Autodesk Inventor part; units mm, degrees
ref_plane "YZ Plane" through (0, 0, 0) normal (1, 0, 0) x (0, 1, 0)
ref_plane "XZ Plane" through (0, 0, 0) normal (0, 1, 0) x (-1, 0, 0)
ref_plane "XY Plane" through (0, 0, 0) normal (0, 0, 1) x (1, 0, 0)
sketch "Sketch1" plane through (0, 0, 0) normal (0, 0, 1) x (1, 0, 0)
  circle A0 centre (0, 0) radius 6.94 construction
  circle A1 centre (0, 0) radius 6.93
  point P0 (0, 0)
  dimension "d0" = 0.01
sketch "Sketch1 outline for Extrusion1" plane through (0, 0, 0) normal (0, 0, 1) x (1, 0, 0)
  circle A0 centre (0, 0) radius 6.93
extrude "Extrusion1" add sketch "Sketch1 outline for Extrusion1" against normal blind 20
sketch "Sketch2" plane through (0, 0, 0) normal (1, 0, 0) x (0, 1, 0)
  line L0 (-6.93, -20) -> (6.93, -20) construction
  line L1 (-6.93, 0) -> (6.93, 0) construction
  line L2 (6.93, -20) -> (6.93, -1.5)
  line L3 (6.93, -1.5) -> (5.93, -20)
  line L4 (6.93, -20) -> (5.93, -20)
  line L5 (0, 4) -> (0, -24)
  point P0 (0, 0)
  dimension "d3" = 1.5
  dimension "d4" = 1
sketch "Sketch2 outline for Revolution1" plane through (0, 0, 0) normal (1, 0, 0) x (0, 1, 0)
  line L0 (5.93, -20) -> (6.93, -20)
  line L1 (6.93, -1.5) -> (5.93, -20)
  line L2 (6.93, -20) -> (6.93, -1.5)
revolve "Revolution1" cut sketch "Sketch2 outline for Revolution1" angle 360 about axis through (0, 0, 0) along (0, 0, -1)
sketch "Sketch3" plane through (0, 0, 0) normal (0, 0, 1) x (1, 0, 0)
  circle A0 centre (0, 0) radius 6.93 construction
  circle A1 centre (0, 0) radius 14.43
  dimension "d6" = 7.5
sketch "Sketch3 outline for Extrusion2" plane through (0, 0, 0) normal (0, 0, 1) x (1, 0, 0)
  circle A0 centre (0, 0) radius 14.43
extrude "Extrusion2" add sketch "Sketch3 outline for Extrusion2" along normal blind 1.5
sketch "Sketch4" plane through (0, 0, -20) normal (0, 0, -1) x (-1, 0, 0)
  circle A0 centre (0, 0) radius 5.93 construction
  circle A1 centre (0, 0) radius 4.43
  dimension "d9" = 1.5
sketch "Sketch4 outline for Extrusion3" plane through (0, 0, -20) normal (0, 0, -1) x (-1, 0, 0)
  circle A0 centre (0, 0) radius 4.43
extrude "Extrusion3" cut sketch "Sketch4 outline for Extrusion3" against normal through all
sketch "Sketch5" plane through (0, 0, 0) normal (1, 0, 0) x (0, 1, 0)
  line L0 (-4.43, 1.5) -> (4.43, 1.5) construction
  line L1 (14.43, 1.5) -> (-14.43, 1.5) construction
  line L2 (4.43, 1.5) -> (14.43, 1.5)
  line L3 (14.43, 1.5) -> (14.43, 18.820508)
  line L4 (14.43, 18.820508) -> (4.43, 1.5)
  point P0 (0, 0)
  dimension "d15" = 60
sketch "Sketch5 outline for Extrusion4" plane through (0, 0, 0) normal (1, 0, 0) x (0, 1, 0)
  line L0 (14.43, 18.820508) -> (4.43, 1.5)
  line L1 (14.43, 1.5) -> (14.43, 18.820508)
  line L2 (4.43, 1.5) -> (14.43, 1.5)
extrude "Extrusion4" add sketch "Sketch5 outline for Extrusion4" along normal mid plane 8
ref_plane "Work Plane1" through (0, 4.43, 1.5) normal (0, 0.5, 0.8660254) x (-1, 0, 0)
sketch "Sketch6" plane through (-4, 14.43, 18.820508) normal (0, -0.8660254, 0.5) x (1, 0, 0)
  line L0 (0, -20) -> (0, 0)
  line L1 (0.50115, -8.72775) -> (7.50139, -8.72775)
  line L2 (8, -20) -> (0, -20)
  line L3 (0, -20) -> (0, -8.97775)
  line L4 (0, -8.97775) -> (8, -8.97775)
  line L5 (8, -8.97775) -> (8, -20)
  point P0 (4, -23.514038)
  dimension "d16" = 0.25
sketch "Sketch6 outline for Extrusion5" plane through (-4, 14.43, 18.820508) normal (0, -0.8660254, 0.5) x (1, 0, 0)
  line L0 (0, -20) -> (8, -20)
  line L1 (0, -8.97775) -> (0, -20)
  line L2 (8, -8.97775) -> (0, -8.97775)
  line L3 (8, -20) -> (8, -8.97775)
extrude "Extrusion5" add sketch "Sketch6 outline for Extrusion5" along normal blind 0.5
sketch "Sketch7" plane through (4, 0, 0) normal (1, 0, 0) x (0, 0, -1)
  line L0 (-1.5, 14.43) -> (-18.820508, 14.43) construction
  line L1 (-18.820508, 14.43) -> (-11.045549, 9.941125) construction
  line L2 (-18.820508, 14.43) -> (-14.820508, 14.43)
  line L3 (-18.820508, 14.43) -> (-14.820508, 12.120599)
  line L4 (-14.820508, 14.43) -> (-14.820508, 12.120599)
  point P0 (0, 0)
  dimension "d19" = 4
sketch "Sketch7 outline for Extrusion6" plane through (4, 0, 0) normal (1, 0, 0) x (0, 0, -1)
  line L0 (-18.820508, 14.43) -> (-14.820508, 14.43)
  line L1 (-14.820508, 14.43) -> (-14.820508, 12.120599)
  line L2 (-14.820508, 12.120599) -> (-18.820508, 14.43)
extrude "Extrusion6" cut sketch "Sketch7 outline for Extrusion6" against normal up to surface (8 mm away)
sketch "Sketch8" plane through (0, 0, 0) normal (0, 0, -1) x (-1, 0, 0)
  circle A0 centre (0, 0) radius 14.43 construction
  circle A1 centre (0, 0) radius 6.93 construction
  circle A2 centre (0, 0) radius 14.43
  circle A3 centre (0, 0) radius 15.93
  dimension "d22" = 0
  dimension "d23" = 1.5
sketch "Sketch8 outline for Extrusion7" plane through (0, 0, 0) normal (0, 0, -1) x (-1, 0, 0)
  circle A0 centre (0, 0) radius 15.93
  circle A1 centre (0, 0) radius 14.43
extrude "Extrusion7" add sketch "Sketch8 outline for Extrusion7" against normal blind 10
mirror "Mirror1" about plane through (0, 0, 0) normal (0, 1, 0) of "Extrusion4", "Extrusion5", "Extrusion6"
properties part number "ECoG_holder_3p0"
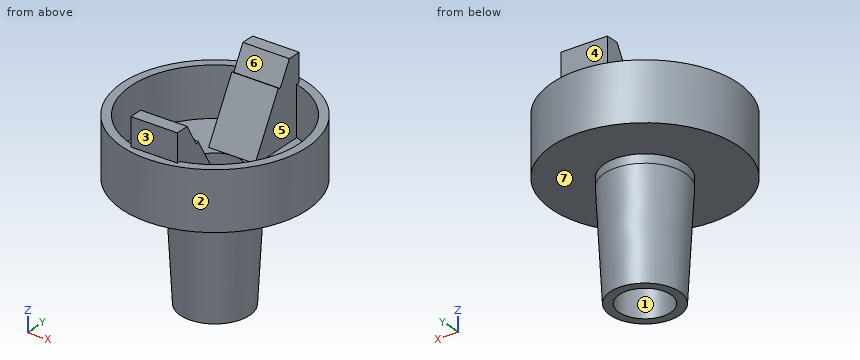
Geometry check sheet. Reference: the model listing, model coordinates, mm. Face numbers are marked on the shaded views. A direction names the side the tool comes from. Give positions to 0.01 mm unless a question says otherwise; leave off trailing zeros. Order: outer loops, then holes, each group sorted by start corner. A loop starts at its lowest first (then second) coordinate and runs counter-clockwise, first axis right, second up. Notation, with made-up numbers: M -35.75,-21.5 L 4.25,-21.5 A31 ccw 4.25,12.5 Z; hole C 34,85 d6. An arc over 180 degrees is marked long. Use a Markdown table: item, result.
Item 1: Tool access check on the marked faces 5, 6 and 7. Record the directions out of +Z, -Z, +X, -X, +Y, -Y that give a thin tool (end or side, any length) a straight path to the whole face; none if there is none.
Answers follow:
| item | result |
|---|---|
| face 5 | +Z |
| face 6 | +Z, +X, -X |
| face 7 | -Z |
Item 2: Material ranges on line 1 along X through (y, z) = (0.5, 5.5); line 2 along X through (y, z) = (-7.5, 4); line 3 along Z through (x, y) = (-3.5, 14.5), recorded low to high.
Answers follow:
| item | result |
|---|---|
| line 1 | x = -15.92 to -14.42, 14.42 to 15.92 |
| line 2 | x = -14.05 to -12.33, -4 to 4, 12.33 to 14.05 |
| line 3 | z = 0 to 10 |
Item 3: Section check B-B (z = 3). Record the cut outline in (x, y).
Answers follow:
| item | result |
|---|---|
| outline | C 0,0 d31.86; hole M -4,-13.86 L -4,-4.72 L 4,-4.72 L 4,-13.86 A14.43 ccw 4,13.86 L 4,4.72 L -4,4.72 L -4,13.86 A14.43 ccw Z |
Item 4: Section check C-C (x = -12). Record the cut outline in (y, z).
Answers follow:
| item | result |
|---|---|
| outline | M -10.48,0 L 10.48,0 L 10.48,10 L 8.01,10 L 8.01,1.5 L -8.01,1.5 L -8.01,10 L -10.48,10 Z |
Item 5: Draft check along Y on the marked faces 1, 2, 3 and 4. Enter one of: +Y half, -Y half, draft (parallel to the pull), parting line (faces both ways), or undercut.
Answers follow:
| item | result |
|---|---|
| face 1 | undercut |
| face 2 | parting line |
| face 3 | -Y half |
| face 4 | +Y half |
Item 6: Section check D-D (y = 10.5). Record the cut outline in (x, z).
Answers follow:
| item | result |
|---|---|
| outline | M -11.98,0 L 11.98,0 L 11.98,10 L 9.9,10 L 9.9,1.5 L 4,1.5 L 4,12.01 L -4,12.01 L -4,1.5 L -9.9,1.5 L -9.9,10 L -11.98,10 Z |
Item 7: Depth check by flat-ended pin: P1, Ø6, axis at y = 8, z = 9.5, coming from the -X side (3 decimals); P2, Ø8.5, axis at y = 8.5, z = 10, coming from the +X side; P3, Ø14, axis at x = 0, y = 0, coming from the +Z side. Enter the tip coordinate at first touch or a pass-through.
Answers follow:
| item | result |
|---|---|
| P1 | stops at x = -15.125 |
| P2 | stops at x = 15.35 |
| P3 | stops at z = 6.95 |
Item 8: Section check A-A (y = 0). Record the cut outline in (x, z).
Answers follow:
| item | result |
|---|---|
| outline | M -15.93,0 L -6.93,0 L -6.93,-1.5 L -5.93,-20 L -4.43,-20 L -4.43,1.5 L -14.43,1.5 L -14.43,10 L -15.93,10 Z; M 4.43,-20 L 5.93,-20 L 6.93,-1.5 L 6.93,0 L 15.93,0 L 15.93,10 L 14.43,10 L 14.43,1.5 L 4.43,1.5 Z |
